from build123d import *

# Parameters (mm, degrees)
F0_W     = 50.8
F0_H     = 76.2
F2_DEPTH = 50.8
F3_W     = 50.8
F3_H     = 76.2
F4_DEPTH = 2.54
F5_T     = -2.54
F6_W     = 50.8
F6_H     = 76.2
F6_W_2   = 45.72
F6_H_2   = 71.12
F6_R     = 11.312852
F7_DEPTH = 3.048


with BuildPart() as f2:
    # F0 (on Front) → F2 (new body)
    with BuildSketch(Plane.XZ):
        Rectangle(F0_W, F0_H)
    extrude(amount=F2_DEPTH)

    # F3 (on Front) → F4 (join)
    with BuildSketch(Plane.XZ):
        Rectangle(F3_W, F3_H)
    extrude(amount=-F4_DEPTH)

    # F5
    f5_openings = [f2.faces().sort_by_distance(p)[0] for p in [
        (0, -50.8, 0),
    ]]
    offset(amount=F5_T, openings=f5_openings)

    # F6 (on offset) → F7 (join)
    with BuildSketch(Plane.XZ.offset(50.8)):
        Rectangle(F6_W, F6_H)
        Rectangle(F6_W_2, F6_H_2, mode=Mode.SUBTRACT)
        Rectangle(F6_W_2, F6_H_2)
        Circle(F6_R, mode=Mode.SUBTRACT)
    extrude(amount=F7_DEPTH)


solid = f2.part
The listing builds one solid part. Answer for the finished solid, in the listing's coordinates (mm). A direction names the side the tool comes from. Give positions to 0.01 mm unless a question says otherwise; leave off trailing zeros. Loops run counter-clockwise (first coordinate to the right, second up) from the corner with the lowest first, then second, coordinate; pieces in that order, holes last. Notation, with made-up numbers: (18, 67) - (56, 67) arc R23 ccw to (56, 90) - close; hole circle Ø1 at (63.25, 87). An arc over 180 degrees is marked (long way). Answer as a JSON object with one key per item and string values.
1. For a pull along X with two mould halves and no side action, classify faces 1 (the cylindrical face through (10.79, -52.3, 3.4)), 2 (the flat face through (-25.4, -25, -1)), 3 (the flat face through (0, -25, -38.1)) as pulls with the +X half, pulls with the -X half, needs draft (parallel to the pull), parting line crosses it, or undercut.
Determined:
{"face 1": "undercut", "face 2": "pulls with the -X half", "face 3": "needs draft"}
2. A flat-ended cylindrical pin translates along its axis: pin 1 Ø8 at (x, z) = (-6.5, 9) entering from -Y. Find the tip coordinate at first contact, or state that the pin passes through.
Determined:
{"pin 1": "y = -53.85"}
3. A cutting plane is placed at B-B (x = 0). Write down the section's boundary in (y, z), then the cut area to 3 significant figures.
Determined:
{"outline": "(-53.85, -38.1) - (2.54, -38.1) - (2.54, 38.1) - (-53.85, 38.1) - (-53.85, 11.31) - (-50.8, 11.31) - (-50.8, 35.56) - (0, 35.56) - (0, -35.56) - (-50.8, -35.56) - (-50.8, -11.31) - (-53.85, -11.31) - close", "area": "615 mm²"}
4. For faces 4 (the flat face through (0, -25, 38.1)), 5 (the flat face through (0, 0, 0)), determine the directions among +Z, -Z, +X, -X, +Y, -Y from which every point of the face is accessible in a straight line to the end or side of a thin tool.
Determined:
{"face 4": "+Z, +X, -X, +Y, -Y", "face 5": "none"}
5. A cutting plane is placed at D-D (z = 0). Write down the section's boundary in (x, y).
Determined:
{"outline": "(-25.4, -53.85) - (-11.31, -53.85) - (-11.31, -50.8) - (-22.86, -50.8) - (-22.86, 0) - (22.86, 0) - (22.86, -50.8) - (11.31, -50.8) - (11.31, -53.85) - (25.4, -53.85) - (25.4, 2.54) - (-25.4, 2.54) - close"}
6. A cutting plane is placed at C-C (y = -33). Write down the section's boundary in (x, z), then the cut area to 3 significant figures.
Determined:
{"outline": "(-25.4, -38.1) - (25.4, -38.1) - (25.4, 38.1) - (-25.4, 38.1) - close; hole (-22.86, -35.56) - (22.86, -35.56) - (22.86, 35.56) - (-22.86, 35.56) - close", "area": "619 mm²"}
7. Find the intervals of material crossed by L1, parallel to X at y = -34.5, z = -13.5; L2, parallel to Z at x = 0, y = -53.1; L3, parallel to Z at x = -12.5, y = -22, in increasing order. Write a range as [from, to].
Determined:
{"L1": "[-25.4, -22.86], [22.86, 25.4]", "L2": "[-38.1, -11.31], [11.31, 38.1]", "L3": "[-38.1, -35.56], [35.56, 38.1]"}
8. A cutting plane is placed at A-A (z = 18). Write down the section's boundary in (x, y).
Determined:
{"outline": "(-25.4, -53.85) - (25.4, -53.85) - (25.4, 2.54) - (-25.4, 2.54) - close; hole (-22.86, -50.8) - (22.86, -50.8) - (22.86, 0) - (-22.86, 0) - close"}
